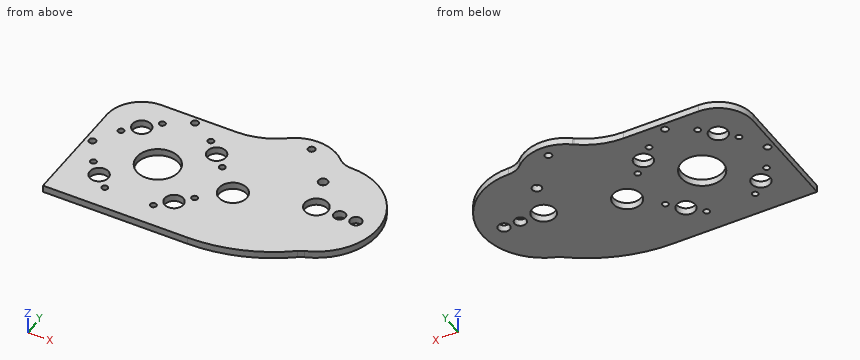
Autodesk Inventor part; units mm, degrees
ref_plane "YZ Plane" through (0, 0, 0) normal (1, 0, 0) x (0, 1, 0)
ref_plane "XZ Plane" through (0, 0, 0) normal (0, 1, 0) x (-1, 0, 0)
ref_plane "XY Plane" through (0, 0, 0) normal (0, 0, 1) x (1, 0, 0)
sketch "スケッチ1" plane through (0, 0, 0) normal (0, 0, 1) x (1, 0, 0)
  line L0 (65.0196, -14.5) -> (65.0196, 33.6804)
  circle A0 centre (80.0196, 33.6804) radius 15 construction
  line L1 (80.0196, 48.6804) -> (112.2, 48.6804)
  circle A1 centre (112.2, 33.6804) radius 15 construction
  line L2 (127.2, -14.5) -> (65.0196, -14.5)
  circle A2 centre (80.0196, 33.6804) radius 3.05 construction
  circle A3 centre (112.2, 33.6804) radius 3.05 construction
  circle A4 centre (112.2, 1.5) radius 3.05 construction
  circle A5 centre (80.0196, 1.5) radius 3.05 construction
  circle A6 centre (96.1098, 17.5902) radius 2.85 construction
  circle A7 centre (128.7687, 16.8502) radius 5.7 construction
  circle A8 centre (160, 25) radius 21.5 construction
  circle A9 centre (128.7687, 16.8502) radius 28.5 construction
  circle A10 centre (128.7687, 16.8502) radius 29.4672 construction
  circle A11 centre (160, 25) radius 25.8772 construction
  circle A12 centre (80.0196, 33.6804) radius 4
  circle A13 centre (112.2, 33.6804) radius 4
  circle A14 centre (80.0196, 1.5) radius 4
  circle A15 centre (112.2, 1.5) radius 4
  arc A16 (112.2, 48.6804) -> (130.0806, 54.5913) centre (112.2, 78.6804) ccw
  arc A17 (153.3164, 53.0826) -> (160, 50.3812) centre (160, 60) ccw
  arc A18 (153.3164, 53.0826) -> (130.0806, 54.5913) centre (140.809, 40.1379) ccw
  circle A19 centre (96.1098, 17.5902) radius 9.025
  circle A20 centre (128.7687, 16.8502) radius 6.025
  circle A21 centre (160, 25) radius 5
  arc A22 (168.6809, 1.1495) -> (160, 50.3812) centre (160, 25) ccw
  arc A23 (168.6809, 1.1495) -> (165.807, -0.5048) centre (171.9707, -7.8892) ccw
  circle A24 centre (171.9707, -7.8892) radius 8.6188 construction
  arc A25 (127.2, -14.5) -> (165.807, -0.5048) centre (127.2, 45.748) ccw
  circle A26 centre (160, 60) radius 8.6188 construction
  circle A27 centre (154.8697, 39.0954) radius 3 construction
  circle A28 centre (154.8697, 39.0954) radius 2
  arc A29 (157.2213, 29.1568) -> (99.1742, 26.079) centre (128.7687, 16.8502) ccw construction
  arc A30 (98.7866, 8.9713) -> (159.6067, 20.0155) centre (128.7687, 16.8502) ccw construction
  arc A31 (80.0196, 48.6804) -> (65.0196, 33.6804) centre (80.0196, 33.6804) ccw
  circle A32 centre (68.0196, 17.5902) radius 1.5
  circle A33 centre (96.1098, 45.6804) radius 1.5
  circle A34 centre (74.3628, 28.0235) radius 1.3
  circle A35 centre (85.6765, 39.3372) radius 1.3
  circle A36 centre (106.5431, 39.3372) radius 1.3
  circle A37 centre (117.8569, 28.0235) radius 1.3
  circle A38 centre (117.8569, 7.1569) radius 1.3
  circle A39 centre (106.5431, -4.1569) radius 1.3
  circle A40 centre (85.6765, -4.1569) radius 1.3
  circle A41 centre (74.3628, 7.1569) radius 1.3
  line L3 (74.3628, 28.0235) -> (85.6765, 39.3372) construction
  line L4 (65.0196, -14.5) -> (65.0196, 33.6804)
  circle A42 centre (80.0196, 33.6804) radius 15 construction
  line L5 (80.0196, 48.6804) -> (112.2, 48.6804)
  circle A43 centre (112.2, 33.6804) radius 15 construction
  line L6 (127.2, -14.5) -> (65.0196, -14.5)
  circle A44 centre (80.0196, 33.6804) radius 3.05 construction
  circle A45 centre (112.2, 33.6804) radius 3.05 construction
  circle A46 centre (112.2, 1.5) radius 3.05 construction
  circle A47 centre (80.0196, 1.5) radius 3.05 construction
  circle A48 centre (96.1098, 17.5902) radius 2.85 construction
  circle A49 centre (128.7687, 16.8502) radius 5.7 construction
  circle A50 centre (160, 25) radius 21.5 construction
  circle A51 centre (128.7687, 16.8502) radius 28.5 construction
  circle A52 centre (128.7687, 16.8502) radius 29.4672 construction
  circle A53 centre (160, 25) radius 25.8772 construction
  circle A54 centre (80.0196, 33.6804) radius 6
  circle A55 centre (112.2, 33.6804) radius 6
  circle A56 centre (80.0196, 1.5) radius 6
  circle A57 centre (112.2, 1.5) radius 6
  arc A58 (112.2, 48.6804) -> (130.5847, 54.9738) centre (112.2, 78.6804) ccw
  arc A59 (154.0473, 53.767) -> (160, 51.3812) centre (160, 60) ccw
  arc A60 (154.0473, 53.767) -> (130.5847, 54.9738) centre (141.6155, 40.7498) ccw
  circle A61 centre (96.1098, 17.5902) radius 9.025
  circle A62 centre (128.7687, 16.8502) radius 6.025
  circle A63 centre (160, 25) radius 2
  arc A64 (169.0229, 0.2098) -> (160, 51.3812) centre (160, 25) ccw
  arc A65 (169.0229, 0.2098) -> (166.7152, -1.0582) centre (171.9707, -7.8892) ccw
  circle A66 centre (171.9707, -7.8892) radius 8.6188 construction
  arc A67 (127.2, -14.5) -> (166.7152, -1.0582) centre (127.2, 50.3027) ccw
  circle A68 centre (160, 60) radius 8.6188 construction
  circle A69 centre (154.8697, 39.0954) radius 3 construction
  circle A70 centre (154.8697, 39.0954) radius 2
  arc A71 (158.348, 26.1273) -> (99.1742, 26.079) centre (128.7687, 16.8502) ccw construction
  arc A72 (98.7866, 8.9713) -> (159.1094, 23.2092) centre (128.7687, 16.8502) ccw construction
  arc A73 (80.0196, 48.6804) -> (65.0196, 33.6804) centre (80.0196, 33.6804) ccw
  circle A74 centre (141.6155, 53.7498) radius 5 construction
  circle A75 centre (141.6155, 53.7498) radius 4
  circle A76 centre (141.6155, 53.7498) radius 1.5
  point P0 (0, 0)
  point P1 (0, 0)
  point P2 (96.1924, 17.5902)
  point P3 (80.1022, 1.5)
  point P4 (112.2826, 1.5)
  point P5 (112.2826, 33.6804)
  point P6 (80.1962, 33.857)
  point P7 (160, 60)
  point P8 (0, 0)
  point P9 (96.1924, 17.5902)
  point P10 (80.1022, 1.5)
  point P11 (112.2826, 1.5)
  point P12 (112.2826, 33.6804)
  point P13 (80.1022, 33.6804)
  point P14 (160, 60)
  point P15 (148.0694, -11.0476)
  point P16 (129.8149, 10.9168)
  point P17 (127.7224, 22.7837)
  point P18 (97.677, 8.7023)
  point P19 (94.5426, 26.4781)
  dimension "d0" = 8
  dimension "d1" = 30
  dimension "d2" = 18.05
  dimension "d3" = 12.05
  dimension "d4" = 10
  dimension "d5" = 1
  dimension "d6" = 18
  dimension "d7" = 4
  dimension "d8" = 31
  dimension "d9" = 32.2772
  dimension "d10" = 60.248
  dimension "d13" = 3
  dimension "d14" = 3
  dimension "d15" = 2.6
  dimension "d16" = 16
  dimension "d25" = 12
  dimension "d26" = 30
  dimension "d27" = 18.05
  dimension "d28" = 12.05
  dimension "d29" = 4
  dimension "d30" = 0
  dimension "d31" = 18
  dimension "d32" = 4
  dimension "d33" = 31
  dimension "d34" = 64.8027
  dimension "d35" = 10
  dimension "d36" = 8
  dimension "d37" = 3
extrude "押し出し1" add sketch "スケッチ1" along normal blind 3 contours L0 A31 L1 A16 A18 A17 A22 A23 A25 L2 | A25 A23 A22 A17 A18 A58 A60 A59 A64 A65 A67 | A54 | A55 | A56 | A57 | A75
sketch "スケッチ2" plane through (0, 0, 0) normal (0, 0, -1) x (-1, 0, 0)
  line L0 (-65.0196, -14.5) -> (-127.2, -14.5)
  line L1 (-65.0196, 33.6804) -> (-65.0196, -14.5)
  arc A0 (-65.0196, 33.6804) -> (-80.0196, 48.6804) centre (-80.0196, 33.6804) ccw
  line L2 (-112.2, 48.6804) -> (-80.0196, 48.6804)
  circle A1 centre (-74.3628, 7.1569) radius 1.3
  circle A2 centre (-106.5431, -4.1569) radius 1.3
  circle A3 centre (-117.8569, 28.0235) radius 1.3
  circle A4 centre (-74.3628, 28.0235) radius 1.3
  circle A5 centre (-68.0196, 17.5902) radius 1.5
  circle A6 centre (-96.1098, 45.6804) radius 1.5
  circle A7 centre (-154.8697, 39.0954) radius 2
  circle A8 centre (-128.7687, 16.8502) radius 6.025
  circle A9 centre (-96.1098, 17.5902) radius 9.025
  circle A10 centre (-112.2, 1.5) radius 4
  circle A11 centre (-80.0196, 1.5) radius 4
  circle A12 centre (-112.2, 33.6804) radius 4
  circle A13 centre (-85.6765, 39.3372) radius 1.3
  circle A14 centre (-106.5431, 39.3372) radius 1.3
  circle A15 centre (-117.8569, 7.1569) radius 1.3
  circle A16 centre (-85.6765, -4.1569) radius 1.3
  circle A17 centre (-160, 25) radius 5
  circle A18 centre (-80.0196, 33.6804) radius 4
  circle A19 centre (-170, 25) radius 2.5
  circle A20 centre (-177, 25) radius 2.5
  line L3 (-160, 25) -> (-180.4045, 25) construction
  arc A21 (-166.7152, -1.0582) -> (-127.2, -14.5) centre (-127.2, 50.3027) ccw
  arc A22 (-130.5847, 54.9738) -> (-154.0473, 53.767) centre (-141.6155, 40.7498) ccw
  arc A23 (-160, 51.3812) -> (-154.0473, 53.767) centre (-160, 60) ccw
  arc A24 (-160, 51.3812) -> (-169.0229, 0.2098) centre (-160, 25) ccw
  arc A25 (-166.7152, -1.0582) -> (-169.0229, 0.2098) centre (-171.9707, -7.8892) ccw
  arc A26 (-130.5847, 54.9738) -> (-112.2, 48.6804) centre (-112.2, 78.6804) ccw
  point P0 (0, 0)
  dimension "d20" = 10
  dimension "d21" = 7
  dimension "d22" = 5
extrude "押し出し2" cut sketch "スケッチ2" against normal blind 10 contours A19 | A20
properties part number "中間フレーム" material "アルミニウム 7075"
Part model, mm, in its own coordinate system. Give positions to 0.01 mm unless a question says otherwise; leave off trailing zeros. Order: outer loops, then holes, each group sorted by start corner. A loop starts at its lowest first (then second) coordinate and runs counter-clockwise, first axis right, second up. Notation, with made-up numbers: (34.25, 6) -> (88.25, 6) arc R22 cw to (88.25, 39) -> close; hole circle Ø2 at (-21.5, 23.25). An arc over 180 degrees is marked (long way). Use one line per item in the form item = value.
(1) Flat gauge pin, fed straight in: P1, Ø1, axis at y = 28.5, z = 2, coming from the +X side. Where does the tip first touch, or does it go through?
Solution:
P1 = 186.21
(2) Saw through at C-C (y = 31.5). Write the cut outline in (x, z).
Solution:
outline = (65.02, 0) -> (76.67, 0) -> (76.67, 3) -> (65.02, 3) -> close; (83.37, 0) -> (108.85, 0) -> (108.85, 3) -> (83.37, 3) -> close; (115.55, 0) -> (185.57, 0) -> (185.57, 3) -> (115.55, 3) -> close
(3) Saw through at D-D (x = 92). Write the cut outline in (y, z), then the cut area to 3 significant figures.
Solution:
outline = (-14.5, 0) -> (9.56, 0) -> (9.56, 3) -> (-14.5, 3) -> close; (25.63, 0) -> (48.68, 0) -> (48.68, 3) -> (25.63, 3) -> close
area = 141 mm²
(4) Saw through at B-B (z = 2.5). Count the separate pieces of the cut face and the enclosed holes in it, then the cut area to 3 significant figures.
Solution:
separate_pieces = 1
enclosed_holes = 21
area = 6,460 mm²
(5) Drill centre lines: line 1 (Y direction, x = 156, z = 1.6); line 2 (X direction, y = 23, z = 1.8); line 3 (Y direction, x = 118, z = 2.5). Where is each one in solid material? Low to high. Write a range as from..to.
Solution:
line_1 = -7.75..22, 28..37.45, 40.75..52.37
line_2 = 65.02..88.89, 103.33..155.42, 164.58..168.5, 171.5..175.5, 178.5..186.31
line_3 = -14.5..5.86, 8.45..26.73, 29.32..49.25
(6) Saw through at A-A (x = 177). Write the cut outline in (y, z).
Solution:
outline = (4.83, 0) -> (22.5, 0) -> (22.5, 3) -> (4.83, 3) -> close; (27.5, 0) -> (45.17, 0) -> (45.17, 3) -> (27.5, 3) -> close
